```python
from build123d import *

# Parameters (mm, degrees)
F0_R     = 6.25
F0_R_2   = 5.1
F1_DEPTH = 25
F2_R     = 10
F3_R     = 8
F4_DEPTH = 200


# Not quite as in the source:
# - a feature names something its author has since deleted; it is built from what else it names


with BuildPart() as f1:
    # F0 (on Top) → F1 (new body)
    with BuildSketch(Plane.XY):
        with BuildLine():
            ThreePointArc((-1.8786394122, 86.9422913227), (-42.1479963116, 19.0841411618), (-60.6516929848, -57.622852377))
            Line((-60.6516929848, -57.622852377), (-123.4119589646, -52.1320405839))
            ThreePointArc((-123.4119589646, -52.1320405839), (-105.3496683323, 30.162565727), (-66.9193045914, 105.1409340308))
            Line((-66.9193045914, 105.1409340308), (-126.574214908, 121.8326206187))
            Line((-126.574214908, 121.8326206187), (-180.4652056167, -70.7699783265))
            Line((-180.4652056167, -70.7699783265), (12.1373933285, -124.6609690352))
            Line((12.1373933285, -124.6609690352), (66.0283840372, 67.9416299099))
            Line((66.0283840372, 67.9416299099), (-1.8786394122, 86.9422913227))
        make_face()
        with Locations((3.3399020095, -25.7191242051)):
            Circle(F0_R, mode=Mode.SUBTRACT)
        with Locations((3.3399020095, -5.7191242051)):
            Circle(F0_R_2, mode=Mode.SUBTRACT)
    extrude(amount=F1_DEPTH)

    # F2
    f2_edges = [f1.edges().sort_by_distance(p)[0] for p in [
        (-123.411959, -52.132041, 12.5),
        (-60.651693, -57.622852, 12.5),
    ]]
    fillet(f2_edges, radius=F2_R)

    # F3 (on face) → F4 (cut, through all)
    with BuildSketch(Plane(origin=(-148.998349815, 41.6903444163, 0), x_dir=(-0.2694549535, -0.9630129947, 0), z_dir=(-0.9630129947, 0.2694549535, 0))):
        with Locations((-63.2203476394, 12.5)):
            Circle(F3_R)
    extrude(amount=-F4_DEPTH, mode=Mode.SUBTRACT)


solid = f1.part
```
CAD build for the part. Positions are in the model's coordinates, mm. A direction names the side the tool comes from. Round coordinates to 2 decimals unless told otherwise and drop trailing zeros. Write each loop counter-clockwise with the first axis right and the second up, starting at its lowest first coordinate (ties: lowest second). Pieces come first, ordered by that corner, then holes. Notation, with made-up numbers: (23, 68) -> (51, 68) arc R17 ccw to (51, 76) -> close; hole circle Ø11 at (-30.75, 17.5). An arc over 180 degrees is marked (long way). Answer in a Markdown table with one row per item. Add a question column.
Item 1: Saw through at D-D, the plane x = -139. Write the cut outline in (y, z).
Item 2: Saw through at A-A, the plane z = 16.25. Write the cut outline in (x, y).
Item 3: Drill centre lines: line 1 (Z direction, x = 43.5, y = 53); line 2 (Y direction, x = -100, z = 12.75); line 3 (Y direction, x = -86, z = 19.75). Where is each one in solid material? Low to high. Write a range as from..to.
Item 4: Drop flat-ended pins along their axis: pin 1 Ø3 at (x, z) = (3, 5.5) entering from +Y; pin 2 Ø12 at (y, z) = (59, 6) entering from +X; pin 3 Ø12 at (y, z) = (-63.5, 22) entering from +X. Give the stop position or say it passes through.
Item 5: Saw through at C-C, the plane y = -100.5. Write the cut outline in (x, z), then the cut area to 3 significant figures.
Item 6: Mould opens along Y. For faces 1 (the face through (-120.11, -49.45, 12.68)), 2 (the face through (-32, 0, 25)), 3 (the face through (-153.142, 26.88, 12.325)) say: pulls with the +Y half, pulls with the -Y half, needs draft (parallel to the pull), parting line crosses it, or undercut.
Item 7: Saw through at B-B, the plane x = -105.5. Count the separate pieces of the cut face and the enclosed holes in it, then the cut area to 3 significant figures.
Item 8: Which spindle directions (+Z, -Z, +X, -X, +Y, -Y) get a long thin tool onto all of the face, cutting with end or side? Do faces 4 (the face through (-91.56, -54.92, 12.32)), 5 (the face through (-39.88, 24.49, 12.32)), 6 (the face through (-102.227, 102.551, 12.852)). Say none if no direction does.
Findings below:
| question | item | result |
|---|---|---|
| 1 | outline | (-82.37, 0) -> (77.42, 0) -> (77.42, 25) -> (-82.37, 25) -> close |
| 2 | outline | (-180.47, -70.77) -> (12.14, -124.66) -> (58.74, 41.88) -> (-18.91, 63.6) arc R265 ccw to (-59.64, -48.04) arc R10 cw to (-70.43, -56.77) -> (-113.29, -53.02) arc R10 cw to (-122.35, -41.87) arc R328 cw to (-81.89, 81.22) -> (-133.87, 95.77) -> close; (-130.06, 109.38) -> (-74.38, 93.8) arc R328 cw to (-66.92, 105.14) -> (-126.57, 121.83) -> close; (-10.42, 75.9) -> (62.54, 55.49) -> (66.03, 67.94) -> (-1.88, 86.94) arc R265 ccw to start; hole circle Ø12.5 at (3.34, -25.72); hole circle Ø10.2 at (3.34, -5.72) |
| 3 | line 1 | z = 0..4.51, 20.49..25 |
| 3 | line 2 | y = -93.28..-54.18, 44.06..85.33, 101.93..114.4 |
| 3 | line 3 | y = -97.2..-55.41, 73.77..86.2, 93.22..110.48 |
| 4 | pin 1 | stops at y = 86 |
| 4 | pin 2 | stops at x = 65.21 |
| 4 | pin 3 | stops at x = 30.93 |
| 5 | outline | (-74.21, 0) -> (18.9, 0) -> (18.9, 25) -> (-74.21, 25) -> close |
| 5 | area | 2,330 mm^2 |
| 6 | face 1 | undercut |
| 6 | face 2 | needs draft |
| 6 | face 3 | pulls with the +Y half |
| 7 | separate pieces | 2 |
| 7 | enclosed holes | 1 |
| 7 | area | 2,900 mm^2 |
| 8 | face 4 | +Z, -Z |
| 8 | face 5 | +Z, -Z, +Y |
| 8 | face 6 | none |
